The drawing under review shows one solid part. Ordinate dimensions are in mm from its lowest x, y, z. Round coordinates to 2 decimals unless told otherwise and drop trailing zeros. Order: outer loops, then holes, each group sorted by start corner. A loop starts at its lowest first (then second) coordinate and runs counter-clockwise, first axis right, second up. Notation, with made-up numbers: (-26.5, 88.25) - (-11.5, 88.25) arc R21 ccw to (-11.5, 119.25) - close; hole circle Ø11 at (-22.75, 42). An arc over 180 degrees is marked (long way). One line per question, with ' | ' between items.
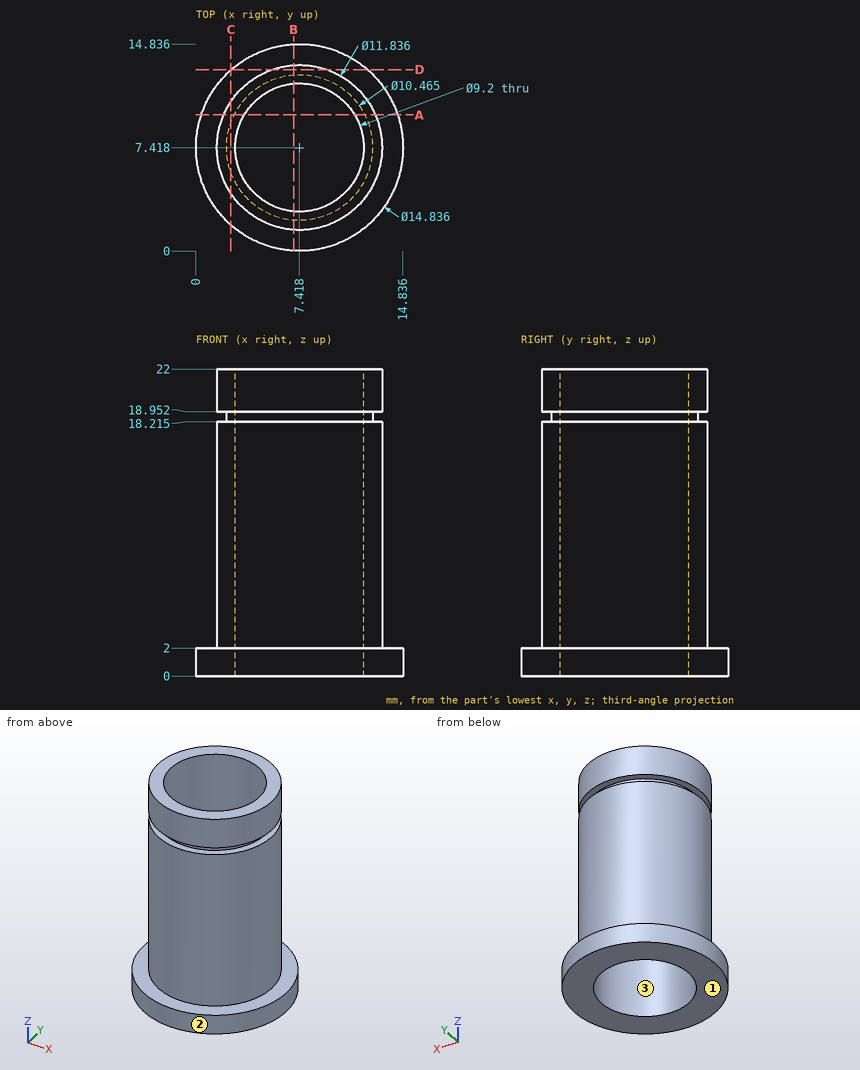
(1) For probe 1 along X at (y, z) = (7.25, 1) (1 decimal); probe 2 along X at (y, z) = (7.25, 5.75) (1 decimal); probe 3 along Y at (x, z) = (7.75, 14.75), list the stretches that pass through material, from the lowest coordinate up. Write a range as [from, to].
Output values:
probe 1: [0, 2.8], [12, 14.8] | probe 2: [1.5, 2.8], [12, 13.3] | probe 3: [1.51, 2.83], [12.01, 13.33]
(2) We need section B-B on x = 7. State the section outline as (y, z) points (1 decimal).
Output values:
outline: (0, 0) - (2.8, 0) - (2.8, 22) - (1.5, 22) - (1.5, 19) - (2.2, 19) - (2.2, 18.2) - (1.5, 18.2) - (1.5, 2) - (0, 2) - close; (12, 0) - (14.8, 0) - (14.8, 2) - (13.3, 2) - (13.3, 18.2) - (12.6, 18.2) - (12.6, 19) - (13.3, 19) - (13.3, 22) - (12, 22) - close
(3) We need section C-C on x = 2.5. State the section outline as (y, z) points (1 decimal), plus the area to 3 significant figures.
Output values:
outline: (1.9, 0) - (13, 0) - (13, 2) - (10.7, 2) - (10.7, 18.2) - (9.2, 18.2) - (9.2, 19) - (10.7, 19) - (10.7, 22) - (4.1, 22) - (4.1, 19) - (5.6, 19) - (5.6, 18.2) - (4.1, 18.2) - (4.1, 2) - (1.9, 2) - close | area: 152 mm^2
(4) We need section D-D on y = 13. State the section outline as (x, z) points (1 decimal).
Output values:
outline: (2.5, 0) - (12.3, 0) - (12.3, 2) - (9.4, 2) - (9.4, 18.2) - (5.5, 18.2) - (5.5, 2) - (2.5, 2) - close; (5.5, 19) - (9.4, 19) - (9.4, 22) - (5.5, 22) - close
(5) We need section A-A on y = 9.75. State the section outline as (x, z) points (1 decimal).
Output values:
outline: (0.4, 0) - (3.5, 0) - (3.5, 22) - (2, 22) - (2, 19) - (2.7, 19) - (2.7, 18.2) - (2, 18.2) - (2, 2) - (0.4, 2) - close; (11.4, 0) - (14.5, 0) - (14.5, 2) - (12.9, 2) - (12.9, 18.2) - (12.1, 18.2) - (12.1, 19) - (12.9, 19) - (12.9, 22) - (11.4, 22) - close
(6) Insertion check: pin 1 (1.5 mm diameter, centred on x = 6, y = 10.5, fed in from -Z); pin 2 (6 mm diameter, centred on x = 6.5, z = 10.5, fed in from -Y); pin 3 (1.5 mm diameter, centred on x = 4.5, z = 11.5, fed in from +Y) (1 decimal); pin 4 (6 mm diameter, centred on x = 7, z = 11, fed in from +Y). Each pin has a flat end and moves straight along its axis. Give the tip position at first contact, or say it passes through.
Output values:
pin 1: through | pin 2: y = 1.5 | pin 3: y = 12.9 | pin 4: y = 13.34
(7) Mouldability with a two-part tool opening along Y and no side actions: class the marked faces 1, 2 and 3 as released by +Y, released by -Y, zero draft, split by the parting line, or undercut.
Output values:
face 1: zero draft | face 2: split by the parting line | face 3: undercut
